Design review of the part built by this model. Coordinates are the model's own, in mm. Face numbers are marked on the shaded views. A direction names the side the tool comes from. Round coordinates to 2 decimals unless told otherwise and drop trailing zeros. Loops run counter-clockwise (first coordinate to the right, second up) from the corner with the lowest first, then second, coordinate; pieces in that order, holes last. Notation, with made-up numbers: (16.25, -29.5) - (32.25, -29.5) arc R10 ccw to (32.25, -17.5) - close; hole circle Ø11 at (23.5, 16.25). An arc over 180 degrees is marked (long way). Answer as CSV lines item,"result". Start each with the question number.
(1) Consider section C-C (x = 12). Give the boundary of the cut face in (y, z) (3 decimals).
(2) Wall thickness on L1, parallel to X at y = 8.25, z = -6.25 (1 decimal); L2, parallel to Y at x = 15.75, z = 0; L3, parallel to Y at x = 21.25, z = 0: over which ranges is each line inside the solid? List them lowest first.
(3) For the marked faces 4, 5 and 6, list the 3-axis set-ups (+Z, -Z, +X, -X, +Y, -Y) from which the entire face can be reached by the end or side of a thin tool; tool diameter is ignored.
(4) For P1, Ø1, axis at y = 2, z = 6.5, coming from the +X side; P2, Ø1, axis at x = 9, z = -3.5, coming from the +Y side; P3, Ø7, axis at y = 0, z = 0, coming from the +X side; P4, Ø1.5, axis at x = 11, z = -1, coming from the +Y side, all flat-tipped, find the tip position at first contact; note any pin that passes through.
(5) Consider section A-A (y = -1.5). Give the boundary of the cut face in (x, z) (1 decimal), and give its area (3 significant figures).
(6) Mouldability with a two-part tool opening along Z and no side actions: class the marked faces 1, 2 and 3 as released by +Z, released by -Z, zero draft, split by the parting line, or undercut.
(7) Consider section B-B (z = -10.75). Give the boundary of the cut face in (x, y) (1 decimal), and give its area (3 significant figures).
(8) Consider section D-D (z = -4.5). Give the boundary of the cut face in (x, y) (1 decimal).
Autodesk Inventor part; units mm, degrees
ref_plane "YZ Plane" through (0, 0, 0) normal (1, 0, 0) x (0, 1, 0)
ref_plane "XZ Plane" through (0, 0, 0) normal (0, 1, 0) x (-1, 0, 0)
ref_plane "XY Plane" through (0, 0, 0) normal (0, 0, 1) x (1, 0, 0)
sketch "Sketch1" plane through (0, 0, 0) normal (1, 0, 0) x (0, 1, 0)
  circle A0 centre (0, 0) radius 12.7
  circle A1 centre (0, 0) radius 4
  dimension "d0" = 25.4
  dimension "d9" = 8
extrude "Extrusion1" add sketch "Sketch1" along normal blind 1.5875
sketch "Sketch2" plane through (1.5875, 0, 0) normal (1, 0, 0) x (0, 0, -1)
  circle A0 centre (0, 0) radius 9.525
  circle A1 centre (0, 0) radius 4
  dimension "d4" = 19.05
extrude "Extrusion2" add sketch "Sketch2" along normal blind 12.7
sketch "Sketch3" plane through (14.2875, 0, 0) normal (1, 0, 0) x (0, 0, -1)
  circle A0 centre (0, 0) radius 12.7
  circle A1 centre (0, 0) radius 4
extrude "Extrusion3" add sketch "Sketch3" along normal blind 1.5875
sketch "Sketch4" plane through (15.875, 0, 0) normal (1, 0, 0) x (0, 0, -1)
  circle A0 centre (0, 0) radius 6.35
  circle A1 centre (0, 0) radius 4
  dimension "d10" = 12.7
extrude "Extrusion4" add sketch "Sketch4" along normal blind 9.525
properties part number "12T XL Pulley"
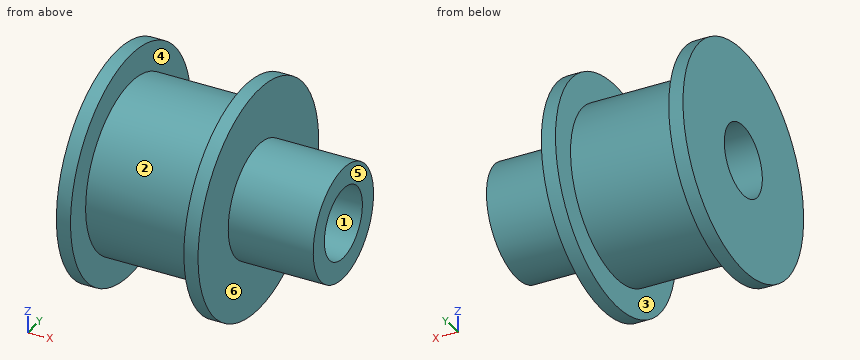
Determined:
1,outline,"circle Ø19.05 at (0, 0); hole circle Ø8 at (0, 0)"
2,L1,"x = 0 to 1.6, 14.3 to 15.9"
2,L2,"y = -12.7 to -4, 4 to 12.7"
2,L3,"y = -6.35 to -4, 4 to 6.35"
3,face 4,"none"
3,face 5,"+Z, -Z, +X, +Y, -Y"
3,face 6,"+X"
4,P1,"stops at x = 25.4"
4,P2,"stops at y = 9.04"
4,P3,"passes through"
4,P4,"stops at y = 9.52"
5,outline,"(0, -12.6) - (1.6, -12.6) - (1.6, -9.4) - (14.3, -9.4) - (14.3, -12.6) - (15.9, -12.6) - (15.9, -6.2) - (25.4, -6.2) - (25.4, -3.7) - (0, -3.7) - close; (0, 3.7) - (25.4, 3.7) - (25.4, 6.2) - (15.9, 6.2) - (15.9, 12.6) - (14.3, 12.6) - (14.3, 9.4) - (1.6, 9.4) - (1.6, 12.6) - (0, 12.6) - close"
5,area,"248 mm^2"
6,face 1,"undercut"
6,face 2,"split by the parting line"
6,face 3,"zero draft"
7,outline,"(0, -6.8) - (1.6, -6.8) - (1.6, 6.8) - (0, 6.8) - close; (14.3, -6.8) - (15.9, -6.8) - (15.9, 6.8) - (14.3, 6.8) - close"
7,area,"42.9 mm^2"
8,outline,"(0, -11.9) - (1.6, -11.9) - (1.6, -8.4) - (14.3, -8.4) - (14.3, -11.9) - (15.9, -11.9) - (15.9, -4.5) - (25.4, -4.5) - (25.4, 4.5) - (15.9, 4.5) - (15.9, 11.9) - (14.3, 11.9) - (14.3, 8.4) - (1.6, 8.4) - (1.6, 11.9) - (0, 11.9) - close"
